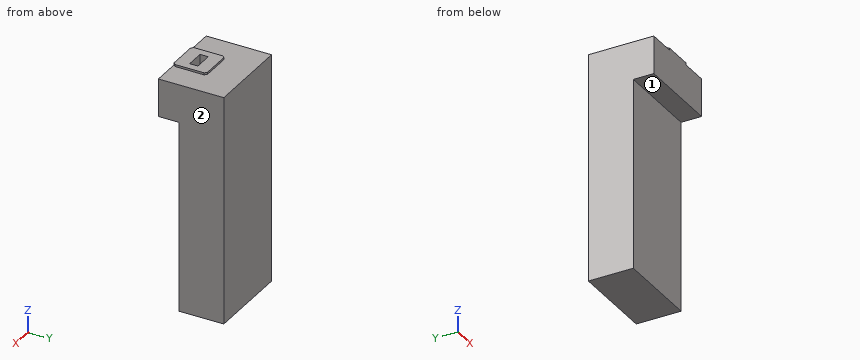
from build123d import *

# Parameters (mm, degrees)
SKETCH1_W           = 111.5
SKETCH1_H           = 31.9
BOSS_EXTRUDE1_DEPTH = 41.3
SKETCH2_W           = 93
SKETCH2_H           = 10
CUT_EXTRUDE1_DEPTH  = 124.10787952
SKETCH3_W           = 16.26
SKETCH3_H           = 16.26
BOSS_EXTRUDE2_DEPTH = 1
SKETCH4_W           = 9
SKETCH4_H           = 4
CUT_EXTRUDE2_DEPTH  = 15
CHAMFER1_SIZE       = 1


with BuildPart() as part:
    # Sketch1 → Boss-Extrude1 (new body)
    with BuildSketch(Plane(origin=(0, 0, 0), x_dir=(0, 0, -1), z_dir=(1, 0, 0))):
        with Locations((55.75, 15.95)):
            Rectangle(SKETCH1_W, SKETCH1_H)
    extrude(amount=-BOSS_EXTRUDE1_DEPTH)

    # Sketch2 → Cut-Extrude1 (cut, through all)
    with BuildSketch(Plane(origin=(0, 0, 0), x_dir=(0, 0, -1), z_dir=(1, 0, 0))):
        with Locations((65, 5)):
            Rectangle(SKETCH2_W, SKETCH2_H)
    extrude(amount=-CUT_EXTRUDE1_DEPTH, mode=Mode.SUBTRACT)

    # Sketch3 → Boss-Extrude2 (add)
    with BuildSketch(Plane.XY):
        with Locations((-20.65, 8.13)):
            Rectangle(SKETCH3_W, SKETCH3_H)
    extrude(amount=BOSS_EXTRUDE2_DEPTH)

    # Sketch4 → Cut-Extrude2 (cut)
    with BuildSketch(Plane.XY.offset(1)):
        with Locations((-20.65, 8.13)):
            Rectangle(SKETCH4_W, SKETCH4_H)
    extrude(amount=-CUT_EXTRUDE2_DEPTH, mode=Mode.SUBTRACT)

    # Chamfer1
    chamfer1_edges = [part.edges().sort_by_distance(p)[0] for p in [
        (-12.52, 0, 0.5),
        (-12.52, 16.26, 0.5),
        (-28.78, 16.26, 0.5),
        (-28.78, 0, 0.5),
    ]]
    chamfer(chamfer1_edges, length=CHAMFER1_SIZE)


solid = part.part
Geometry: final body of the model. Coordinates: model frame, mm. Face numbers are marked on the shaded views. A direction names the side the tool comes from. Give positions to 0.01 mm unless a question says otherwise; leave off trailing zeros. Loops run counter-clockwise (first coordinate to the right, second up) from the corner with the lowest first, then second, coordinate; pieces in that order, holes last. Notation, with made-up numbers: (38, 65.25) - (54, 65.25) arc R15 ccw to (54, 80.25) - close; hole circle Ø8 at (-19, -19.75). An arc over 180 degrees is marked (long way). Answer as CSV lines item,"result". Start each with the question number.
1. Pin query (flat end, axial travel): P1, Ø0.5, axis at y = 7, z = 0.5, coming from the +X side; P2, Ø3, axis at x = -30, y = 3.5, coming from the -Z side; P3, Ø4, axis at x = -10.5, y = 22.5, coming from the +Z side. Return the tip coordinate at first contact, or that it passes through.
2. Section B-B, the plane y = 8. Return loops of the section in (x, z), plus the area to 3 significant figures.
3. Section D-D, the plane x = -34.5. Return loops of the section in (y, z), plus the area to 3 significant figures.
4. Section A-A, the plane x = -21.5. Return loops of the section in (y, z), plus the area to 3 significant figures.
5. Reachability of the marked faces 1 and 2 from +Z, -Z, +X, -X, +Y, -Y: full face, straight path, thin tool, end or side. Return the list, or none.
6. Section C-C, the plane z = -48. Return loops of the section in (x, y).
7. Ray query, L1, parallel to Z at x = -37, y = 2; L2, parallel to Y at x = -22, z = -24; L3, parallel to Z at x = -7.5, y = 19.5. Return the intervals inside material, ascending.
Answers:
1,P1,"stops at x = -12.52"
1,P2,"stops at z = -18.5"
1,P3,"stops at z = 0"
2,outline,"(-41.3, -18.5) - (0, -18.5) - (0, 0) - (-12.52, 0) - (-12.52, 1) - (-16.15, 1) - (-16.15, -14) - (-25.15, -14) - (-25.15, 1) - (-28.78, 1) - (-28.78, 0) - (-41.3, 0) - close"
2,area,"645 mm2"
3,outline,"(0, -18.5) - (10, -18.5) - (10, -111.5) - (31.9, -111.5) - (31.9, 0) - (0, 0) - close"
3,area,"2,630 mm2"
4,outline,"(0, -18.5) - (10, -18.5) - (10, -111.5) - (31.9, -111.5) - (31.9, 0) - (16.26, 0) - (16.26, 1) - (10.13, 1) - (10.13, -14) - (6.13, -14) - (6.13, 1) - (0, 1) - close"
4,area,"2,580 mm2"
5,face 1,"-Z, +X, -X, -Y"
5,face 2,"+Z, -Z, +X, +Y, -Y"
6,outline,"(-41.3, 10) - (0, 10) - (0, 31.9) - (-41.3, 31.9) - close"
7,L1,"z = -18.5 to 0"
7,L2,"y = 10 to 31.9"
7,L3,"z = -111.5 to 0"
